```python
from build123d import *

# Parameters (mm, degrees)
SKETCH001_R  = 1
PAD_DEPTH    = 3.5
SKETCH002_R  = 0.5
POCKET_DEPTH = 10


with BuildPart() as part:
    # Sketch001 → Pad (new body)
    with BuildSketch(Plane.XY):
        Polygon((9, 0), (9, 15), (0, 15), (0, 40), (50, 40), (50, 15), (41, 15), (41, 0), (31, 0), (31, 25), (19, 25), (19, 0), align=None)
        with Locations((46.504002, 36.501442)):
            Circle(SKETCH001_R, mode=Mode.SUBTRACT)
        with Locations((3.500559, 36.501442)):
            Circle(SKETCH001_R, mode=Mode.SUBTRACT)
        with Locations((3.500559, 18.503159)):
            Circle(SKETCH001_R, mode=Mode.SUBTRACT)
        with Locations((46.496666, 18.503159)):
            Circle(SKETCH001_R, mode=Mode.SUBTRACT)
    extrude(amount=PAD_DEPTH)

    # Sketch002 (on Face9 of Pad) → Pocket (cut)
    with BuildSketch(Plane.XZ):
        with Locations((38.501091, 1.746948)):
            Circle(SKETCH002_R)
        with Locations((33.500816, 1.749735)):
            Circle(SKETCH002_R)
        with Locations((16.500931, 1.75016)):
            Circle(SKETCH002_R)
        with Locations((11.498322, 1.75016)):
            Circle(SKETCH002_R)
    extrude(amount=-POCKET_DEPTH, mode=Mode.SUBTRACT)


solid = part.part
```
Verification items for the finished model (mm, model axes). A direction names the side the tool comes from. Give positions to 0.01 mm unless a question says otherwise; leave off trailing zeros. Loops run counter-clockwise (first coordinate to the right, second up) from the corner with the lowest first, then second, coordinate; pieces in that order, holes last.
1. Section check C-C, the plane x = 29. Enter the section's corners in (y, z), then the cut area to 3 significant figures.
2. Set-up check for faces 5 (the flat face through (5, 15, 2)), 6 (the flat face through (41, 8, 2)), 7 (the flat face through (31, 12, 2)), 8 (the flat face through (33.5, 10, 1.8)), 9 (the flat face through (50, 28, 2)): record each of +Z, -Z, +X, -X, +Y, -Y from which the full face is reachable in a straight line by a thin tool's end or side.
3. Mould release check, pull along Y, two halves, no side actions. Record for faces 1 (the cylindrical face through (47.45, 18.8, 1.73)), 2 (the flat face through (25, 29, 0)), 3 (the flat face through (25, 40, 2)), 4 (the flat face through (46, 15, 2)): released by +Y, released by -Y, zero draft, split by the parting line, or undercut.
4. Go/stop test with flat-tipped pins: pin 1 Ø1.8 at (y, z) = (9, 1.5) entering from -X; pin 2 Ø1.6 at (x, y) = (46.5, 18.5) entering from -Z; pin 3 Ø1.5 at (x, z) = (21, 3) entering from -Y; pin 4 Ø1.8 at (x, z) = (47, 1.5) entering from -Y. Record where each tip stops, or that it passes through.
5. Thickness scan on line 1 (X direction, y = 10.5, z = 1.45); line 2 (Y direction, x = 29, z = 2.15); line 3 (Y direction, x = 43.5, z = 2). Record the ranges inside material, lowest first.
6. Section check A-A, the plane y = 6.5. Enter the section's corners in (x, z).
7. Section check B-B, the plane z = 2.8. Enter the section's corners in (x, y).
Geometry says:
1. outline: (25, 0) - (40, 0) - (40, 3.5) - (25, 3.5) - close
1. area: 52.5 mm2
2. face 5: +Z, -Z, -X, -Y
2. face 6: +Z, -Z, +X, -Y
2. face 7: +Z, -Z, -Y
2. face 8: -Y
2. face 9: +Z, -Z, +X, +Y, -Y
3. face 1: undercut
3. face 2: zero draft
3. face 3: released by +Y
3. face 4: released by -Y
4. pin 1: stops at x = 9
4. pin 2: passes through
4. pin 3: stops at y = 25
4. pin 4: stops at y = 15
5. line 1: x = 9 to 19, 31 to 41
5. line 2: y = 25 to 40
5. line 3: y = 15 to 40
6. outline: (9, 0) - (19, 0) - (19, 3.5) - (9, 3.5) - close; (31, 0) - (41, 0) - (41, 3.5) - (31, 3.5) - close; hole circle Ø1 at (11.5, 1.75); hole circle Ø1 at (16.5, 1.75); hole circle Ø1 at (33.5, 1.75); hole circle Ø1 at (38.5, 1.75)
7. outline: (0, 15) - (9, 15) - (9, 0) - (19, 0) - (19, 25) - (31, 25) - (31, 0) - (41, 0) - (41, 15) - (50, 15) - (50, 40) - (0, 40) - close; hole circle Ø2 at (3.5, 18.5); hole circle Ø2 at (3.5, 36.5); hole circle Ø2 at (46.5, 18.5); hole circle Ø2 at (46.5, 36.5)
